Study the drawing (mm; zero at the part's minimum x, y, z) and answer. Give positions to 0.01 mm unless a question says otherwise; leave off trailing zeros. Order: outer loops, then holes, each group sorted by start corner. A loop starts at its lowest first (then second) coordinate and runs counter-clockwise, first axis right, second up. Notation, with made-up numbers: (2.25, -21) - (27.25, -21) arc R15 cw to (27.25, 5) - close; hole circle Ø4 at (66, 52.25). An arc over 180 degrees is marked (long way). Write each question's results on one line, items separated by ' | '. Start each with the question number.
1. Section C-C (z = 0.75) is taken. Give the vertices of the cut face in (x, y), and give its area (3 significant figures).
2. Section A-A (x = 48.5) is taken. Give the vertices of the cut face in (y, z).
3. Section D-D (x = 55) is taken. Give the vertices of the cut face in (y, z).
4. Find the intervals of material crossed by L1, parallel to Y at x = 48.5, z = 0.3; L2, parallel to X at y = 44.5, z = 0.25; L3, parallel to Y at x = 55, z = 0.65, in increasing order.
5. Section B-B (y = 26) is taken. Give the vertices of the cut face in (x, z), and give its area (3 significant figures).
6. Determine the mould class of the marked faces 1 and 2 for opening direction Z: released by +Z, released by -Z, zero draft, split by the parting line, or undercut.
7. A flat-ended cylindrical pin translates along its axis: pin 1 (4 mm diameter, centred on x = 48.5, y = 3.5, fed in from +Z). Find the tip coordinate at first contact, or state that the pin passes through.
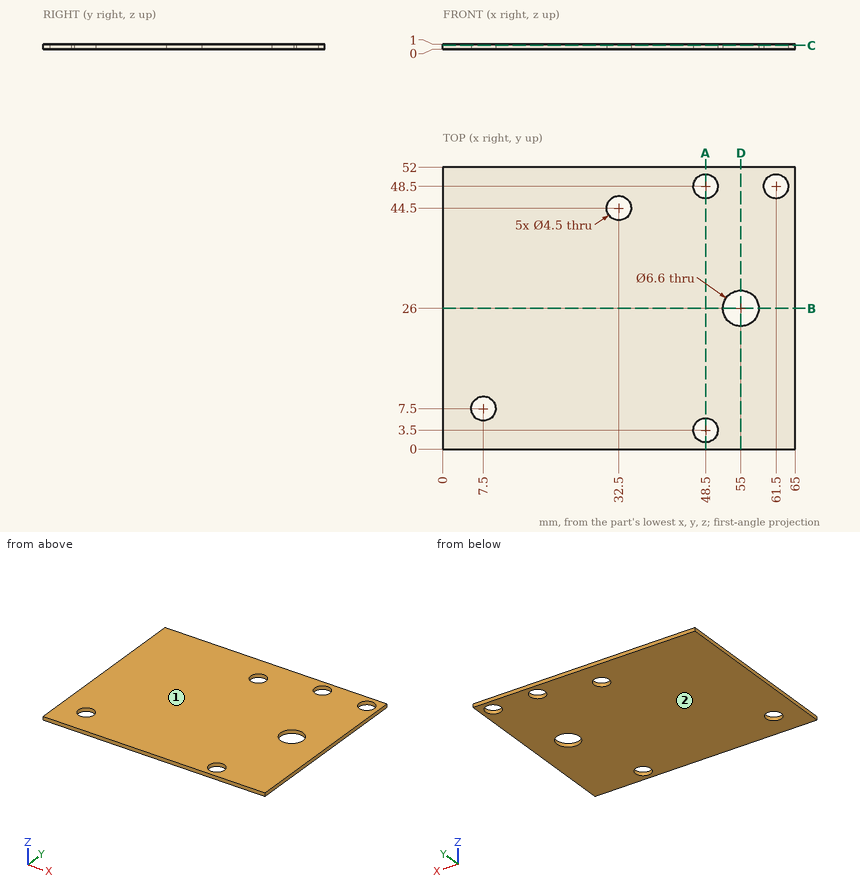
Reported:
1) outline: (0, 0) - (65, 0) - (65, 52) - (0, 52) - close; hole circle Ø4.5 at (7.5, 7.5); hole circle Ø4.5 at (32.5, 44.5); hole circle Ø4.5 at (48.5, 3.5); hole circle Ø4.5 at (48.5, 48.5); hole circle Ø6.6 at (55, 26); hole circle Ø4.5 at (61.5, 48.5) | area: 3,270 mm²
2) outline: (0, 0) - (1.25, 0) - (1.25, 1) - (0, 1) - close; (5.75, 0) - (46.25, 0) - (46.25, 1) - (5.75, 1) - close; (50.75, 0) - (52, 0) - (52, 1) - (50.75, 1) - close
3) outline: (0, 0) - (22.7, 0) - (22.7, 1) - (0, 1) - close; (29.3, 0) - (52, 0) - (52, 1) - (29.3, 1) - close
4) L1: 0 to 1.25, 5.75 to 46.25, 50.75 to 52 | L2: 0 to 30.25, 34.75 to 65 | L3: 0 to 22.7, 29.3 to 52
5) outline: (0, 0) - (51.7, 0) - (51.7, 1) - (0, 1) - close; (58.3, 0) - (65, 0) - (65, 1) - (58.3, 1) - close | area: 58.4 mm²
6) face 1: released by +Z | face 2: released by -Z
7) pin 1: through
